Check sheet for the modelled part. Datum: model origin and axes. Units: mm. A direction names the side the tool comes from. Round coordinates to 2 decimals unless told otherwise and drop trailing zeros. Loops run counter-clockwise (first coordinate to the right, second up) from the corner with the lowest first, then second, coordinate; pieces in that order, holes last. Notation, with made-up numbers: (-6.75, 26.25) -> (42.25, 26.25) arc R20 ccw to (42.25, 37.25) -> close; hole circle Ø11 at (-36, 82.5). An arc over 180 degrees is marked (long way). One line per question, with ' | ' between items.
```python
from build123d import *

# Parameters (mm, degrees)
SKETCH1_W                                      = 36.5
SKETCH1_H                                      = 45
BOSS_EXTRUDE1_DEPTH                            = 6.35
SKETCH4_W                                      = 50
SKETCH4_H                                      = 50
CUT_EXTRUDE1_DEPTH                             = 4
CUT_EXTRUDE2_DEPTH                             = 19
F_2_56_TAPPED_HOLE1_D                          = 1.778
CBORE_FOR_2_SOCKET_HEAD_CAP_SCREW1_D           = 2.7051
CBORE_FOR_2_SOCKET_HEAD_CAP_SCREW1_CBORE_D     = 4.7625
CBORE_FOR_2_SOCKET_HEAD_CAP_SCREW1_CBORE_DEPTH = 2.18439746


with BuildPart() as part:
    # Sketch1 → Boss-Extrude1 (new body)
    with BuildSketch(Plane.XY):
        with Locations((18.25, 22.5)):
            Rectangle(SKETCH1_W, SKETCH1_H)
    extrude(amount=BOSS_EXTRUDE1_DEPTH)

    # Sketch4 → Cut-Extrude1 (cut)
    with BuildSketch(Plane(origin=(-4.216220414, 1.201768304, -5.904135163), x_dir=(-0.816779309, -0.191151006, 0.544364633), z_dir=(-0.573332653, 0.16341959, -0.802859705))):
        with Locations((-8.601795261, 43.553754656)):
            Rectangle(SKETCH4_W, SKETCH4_H)
    extrude(amount=-CUT_EXTRUDE1_DEPTH, mode=Mode.SUBTRACT)

    # Sketch7 → Cut-Extrude2 (cut)
    with BuildSketch(Plane(origin=(0, 0, 0), x_dir=(-1, 0, 0), z_dir=(0, 0, -1))):
        with BuildLine():
            Line((0, 0), (-13, 0))
            Line((-13, 0), (-13, 29.6625))
            ThreePointArc((-13, 29.6625), (-12.535032015, 30.785032015), (-11.4125, 31.25))
            Line((-11.4125, 31.25), (0, 31.25))
            Line((0, 31.25), (0, 0))
        make_face()
        with BuildLine():
            Line((-36.5, 0), (-29, 0))
            Line((-29, 0), (-29, 33.4125))
            ThreePointArc((-29, 33.4125), (-29.464967985, 34.535032015), (-30.5875, 35))
            Line((-30.5875, 35), (-36.5, 35))
            Line((-36.5, 35), (-36.5, 0))
        make_face()
        with BuildLine():
            Line((-13, 45), (-13, 41.8375))
            ThreePointArc((-13, 41.8375), (-12.535032015, 40.714967985), (-11.4125, 40.25))
            Line((-11.4125, 40.25), (0, 40.25))
            Line((0, 40.25), (0, 45))
            Line((0, 45), (-13, 45))
        make_face()
    extrude(amount=-CUT_EXTRUDE2_DEPTH, mode=Mode.SUBTRACT)

    # #2-56 Tapped Hole1 (through all)
    with Locations(Plane(origin=(-1.9228898, 0.548089945, -2.692696342), x_dir=(-0.816779309, -0.191151006, 0.544364633), z_dir=(-0.573332653, 0.16341959, -0.802859705))):
        with Locations((-7.966944936, 34.99181106)):
            Hole(F_2_56_TAPPED_HOLE1_D / 2)

    # CBORE for #2 Socket Head Cap Screw1 (through all)
    with Locations(Plane(origin=(0, 0, 0), x_dir=(-1, 0, 0), z_dir=(0, 0, -1))):
        with Locations((-21, 10), (-32, 40)):
            CounterBoreHole(CBORE_FOR_2_SOCKET_HEAD_CAP_SCREW1_D / 2, CBORE_FOR_2_SOCKET_HEAD_CAP_SCREW1_CBORE_D / 2, CBORE_FOR_2_SOCKET_HEAD_CAP_SCREW1_CBORE_DEPTH)


solid = part.part
```
(1) Sectioned sample at D-D, the plane y = 32.5. Record the cut outline in (x, z), and give its area (3 significant figures).
Answer:
outline: (0, 2.44) -> (3.41, 0) -> (29, 0) -> (29, 6.35) -> (0, 6.35) -> close | area: 180 mm2
(2) Sectioned sample at C-C, the plane z = 5.5. Count the separate pieces of the cut face and the enclosed holes in it, and give its area (3 significant figures).
Answer:
separate pieces: 1 | enclosed holes: 3 | area: 899 mm2
(3) Mould release check, pull along Y, two halves, no side actions. Record for faces 1 (the face through (21, 0, 3)), 2 (the face through (2.079, 37.026, 1.875)), 3 (the face through (21, 8, 2.184)), 4 (the face through (33.755, 41.609, 1.077)): +Y half, -Y half, draft (parallel to the pull), parting line (faces both ways), or undercut.
Answer:
face 1: -Y half | face 2: +Y half | face 3: undercut | face 4: undercut
(4) Set-up check for faces 5 (the face through (34, 35, 3)), 6 (the face through (0, 36, 5)), 7 (the face through (36.5, 40, 3)), 8 (the face through (19.9, 7.89, 1.08)), 9 (the face through (13, 15, 3)): record each of +Z, -Z, +X, -X, +Y, -Y from which the full face is reachable in a straight line by a thin tool's end or side.
Answer:
face 5: +Z, -Z, +X, -Y | face 6: +Z, -Z, -X, +Y, -Y | face 7: +Z, -Z, +X, +Y, -Y | face 8: -Z | face 9: +Z, -Z, -X, -Y
(5) Scan lines: probe 1 along Y at (x, z) = (32, 3.1); probe 2 along Y at (x, z) = (32, 1.35); probe 3 along X at (y, z) = (6.5, 4.75). Record each from-to range of solid material in increasing order.
Answer:
probe 1: y = 35 to 38.65, 41.35 to 45 | probe 2: y = 35 to 37.62, 42.38 to 45 | probe 3: x = 13 to 29
(6) Go/stop test with flat-tipped pins: pin 1 (1.8 mm diameter, centred on x = 34.5, z = 4.5, fed in from -Y); pin 2 (4.5 mm diameter, centred on x = 32, y = 40, fed in from -Z); pin 3 (1.9 mm diameter, centred on y = 23, z = 4, fed in from +X). Record where each tip stops, or that it passes through.
Answer:
pin 1: stops at y = 35 | pin 2: stops at z = 2.18 | pin 3: stops at x = 29
(7) Sectioned sample at A-A, the plane x = 32. Record the cut outline in (y, z).
Answer:
outline: (35, 0) -> (37.62, 0) -> (37.62, 2.18) -> (38.65, 2.18) -> (38.65, 6.35) -> (35, 6.35) -> close; (41.35, 2.18) -> (42.38, 2.18) -> (42.38, 0) -> (45, 0) -> (45, 6.35) -> (41.35, 6.35) -> close
(8) Sectioned sample at B-B, the plane y = 10. Record the cut outline in (x, z), and give its area (3 significant figures).
Answer:
outline: (13, 0) -> (18.62, 0) -> (18.62, 2.18) -> (19.65, 2.18) -> (19.65, 6.35) -> (13, 6.35) -> close; (22.35, 2.18) -> (23.38, 2.18) -> (23.38, 0) -> (29, 0) -> (29, 6.35) -> (22.35, 6.35) -> close | area: 79.9 mm2
